```python
from build123d import *

# Parameters (mm, degrees)
CROQUIS1_W                 = 7.5
CROQUIS1_H                 = 6.1
SALIENTE_EXTRUIR2_DEPTH    = 5
CROQUIS2_R                 = 1.6
CORTAR_EXTRUIR1_DEPTH      = 18
REDONDEO1_R                = 1
CORTAR_EXTRUIR2_DEPTH      = 38.482562804
CORTAR_EXTRUIR2_DEPTH_BACK = 38.482562804
CROQUIS3_R                 = 2.1
REDONDEO2_R                = 2


with BuildPart() as part:
    # Croquis1 → Saliente-Extruir2 (new, symmetric)
    # profile 1 of 8: a face of its own
    with BuildSketch(Plane.XY):
        with BuildLine():
            ThreePointArc((12.649110641, 13.5), (6.800735254, 17.204650534), (-1e-09, 18.5))
            ThreePointArc((-1e-09, 18.5), (-6.800735255, 17.204650534), (-12.649110641, 13.5))
            ThreePointArc((-12.649110641, 13.5), (-7.356679045, -16.974371076), (18.5, 0))
            ThreePointArc((18.5, 0), (16.974371076, 7.356679045), (12.649110641, 13.5))
        make_face()
        with BuildLine():
            ThreePointArc((11.05, 0), (-7.813529932, -7.813529932), (0, 11.05))
            ThreePointArc((0, 11.05), (7.813529932, 7.813529932), (11.05, 0))
        make_face(mode=Mode.SUBTRACT)
    # profile 2 of 8: a face of its own
    with BuildSketch(Plane.XY):
        with BuildLine():
            ThreePointArc((12.649110641, 13.5), (6.800735254, 17.204650534), (-1e-09, 18.5))
            ThreePointArc((-1e-09, 18.5), (-6.800735255, 17.204650534), (-12.649110641, 13.5))
            ThreePointArc((-12.649110641, 13.5), (-7.356679045, -16.974371076), (18.5, 0))
            ThreePointArc((18.5, 0), (16.974371076, 7.356679045), (12.649110641, 13.5))
        make_face()
        with BuildLine():
            ThreePointArc((11.05, 0), (-7.813529932, -7.813529932), (0, 11.05))
            ThreePointArc((0, 11.05), (7.813529932, 7.813529932), (11.05, 0))
        make_face(mode=Mode.SUBTRACT)
    # profile 3 of 8: a face of its own
    with BuildSketch(Plane.XY):
        with BuildLine():
            Line((7.5, 18.5), (-1e-09, 18.5))
            ThreePointArc((-1e-09, 18.5), (6.800735254, 17.204650534), (12.649110641, 13.5))
            Line((12.649110641, 13.5), (22.5, 13.5))
            Line((22.5, 13.5), (22.5, 18.5))
            Line((22.5, 18.5), (7.5, 18.5))
        make_face()
    # profile 4 of 8: a face of its own
    with BuildSketch(Plane.XY):
        with BuildLine():
            Line((-7.5, 18.5), (-22.5, 18.5))
            Line((-22.5, 18.5), (-22.5, 13.5))
            Line((-22.5, 13.5), (-12.649110641, 13.5))
            ThreePointArc((-12.649110641, 13.5), (-6.800735255, 17.204650534), (-1e-09, 18.5))
            Line((-1e-09, 18.5), (-7.5, 18.5))
        make_face()
    # profile 5 of 8: a face of its own
    with BuildSketch(Plane.XY):
        Polygon((-22.5, 21.5), (-7.5, 21.5), (-7.5, 24.6), (0, 24.6), (0, 29.558290112), (-22.5, 29.558290112), (-22.5, 24.558290112), align=None)
    # profile 6 of 8: a face of its own
    with BuildSketch(Plane.XY):
        with Locations((3.75, 21.55)):
            Rectangle(CROQUIS1_W, CROQUIS1_H)
    # profile 7 of 8: a face of its own
    with BuildSketch(Plane.XY):
        Polygon((-7.5, 21.5), (-7.5, 18.5), (-1e-09, 18.5), (0, 24.6), (-7.5, 24.6), align=None)
    # profile 8 of 8: a face of its own
    with BuildSketch(Plane.XY):
        Polygon((0, 29.558290112), (0, 24.6), (7.5, 24.6), (22.5, 24.6), (22.5, 29.558290112), align=None)
    extrude(amount=SALIENTE_EXTRUIR2_DEPTH, both=True)

    # Croquis2 → Cortar-Extruir1 (cut)
    with BuildSketch(Plane(origin=(0, 29.558290112, 0), x_dir=(1, 0, 0), z_dir=(0, 1, 0))):
        with Locations(Location((-17.5, 0, 0), (0, 0, 270))):
            Circle(CROQUIS2_R)
        with Locations(Location((17.5, 0, 0), (0, 0, 270))):
            Circle(CROQUIS2_R)
    extrude(amount=-CORTAR_EXTRUIR1_DEPTH, mode=Mode.SUBTRACT)

    # Redondeo1
    redondeo1_edges = [part.edges().sort_by_distance(p)[0] for p in [
        (7.813529932, 7.813529932, 5),
    ]]
    fillet(redondeo1_edges, radius=REDONDEO1_R)

    # Croquis3 → Cortar-Extruir2 (cut, two sides: drawn at the far end of the back side and taken through both)
    with BuildSketch(Plane(origin=(0, 0, 0), x_dir=(0, 0, -1), z_dir=(1, 0, 0)).offset(-CORTAR_EXTRUIR2_DEPTH_BACK)):
        Circle(CROQUIS3_R)
    extrude(amount=CORTAR_EXTRUIR2_DEPTH + CORTAR_EXTRUIR2_DEPTH_BACK, mode=Mode.SUBTRACT)

    # Redondeo2
    redondeo2_edges = [part.edges().sort_by_distance(p)[0] for p in [
        (22.5, 16, -5),
        (-22.5, 16, -5),
        (-22.5, 25.529145056, -5),
        (22.5, 27.079145056, 5),
        (22.5, 27.079145056, -5),
        (-22.5, 25.529145056, 5),
        (-22.5, 16, 5),
        (22.5, 16, 5),
    ]]
    fillet(redondeo2_edges, radius=REDONDEO2_R)


solid = part.part
```
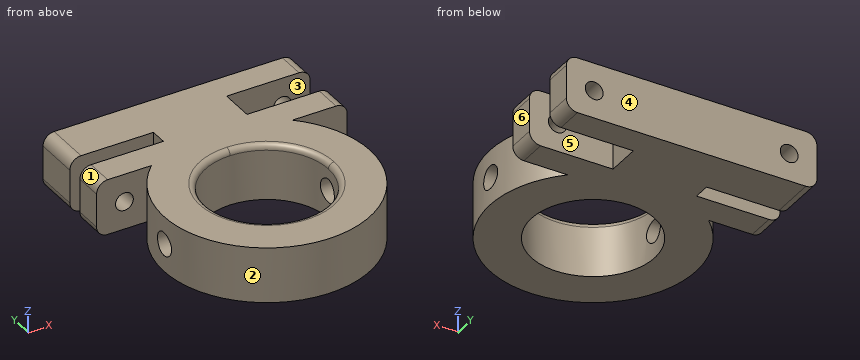
CAD build for the part. Positions are in the model's coordinates, mm. Face numbers are marked on the shaded views. A direction names the side the tool comes from. Give positions to 0.01 mm unless a question says otherwise; leave off trailing zeros. Loops run counter-clockwise (first coordinate to the right, second up) from the corner with the lowest first, then second, coordinate; pieces in that order, holes last. Notation, with made-up numbers: (13, 14) -> (41, 14) arc R18 ccw to (41, 32) -> close; hole circle Ø2 at (81, 67.25). An arc over 180 degrees is marked (long way). Use a Markdown table: item, result.
1. Flat gauge pins, fed straight in: pin 1 (3 mm diameter, centred on y = 22, z = -0.5, fed in from +X); pin 2 (1.5 mm diameter, centred on y = 19.5, z = -2, fed in from -X); pin 3 (5.5 mm diameter, centred on y = 0, z = 0, fed in from +X). Where does each tip first touch, or does it go through?
Check result:
| item | result |
|---|---|
| pin 1 | stops at x = 7.5 |
| pin 2 | stops at x = -7.5 |
| pin 3 | stops at x = 18.5 |
2. Slice it at D-D (z = -1). Give the number of separate pieces and of enclosed holes in the cut face, plus the area to 3 significant figures.
Check result:
| item | result |
|---|---|
| separate pieces | 6 |
| enclosed holes | 0 |
| area | 1,080 mm^2 |
3. Wall check: L1, parallel to Y at x = -13.5, z = 0; L2, parallel to X at y = 16, z = 1; L3, parallel to Y at x = 16, z = 1.5. Give the ranges that are in metal, low to high. Write a range as [from, to].
Check result:
| item | result |
|---|---|
| L1 | y = [-12.65, -2.1], [2.1, 12.65], [13.5, 18.5], [21.5, 29.56] |
| L2 | x = [-22.5, -18.75], [-16.25, 16.25], [18.75, 22.5] |
| L3 | y = [-9.29, -1.47], [1.47, 9.29], [13.5, 18.5], [24.6, 29.56] |
4. Mould opens along Y. For the marked faces 1, 2, 3 and 4 say: pulls with the +Y half, pulls with the -Y half, needs draft (parallel to the pull), parting line crosses it, or undercut.
Check result:
| item | result |
|---|---|
| face 1 | needs draft |
| face 2 | undercut |
| face 3 | undercut |
| face 4 | pulls with the +Y half |
5. Slice it at B-B (x = 17.5). List the corners of the cut face in (y, z).
Check result:
| item | result |
|---|---|
| outline | (-6, -5) -> (6, -5) -> (6, 5) -> (-6, 5) -> close; (13.5, -5) -> (18.5, -5) -> (18.5, -1.6) -> (13.5, -1.6) -> close; (13.5, 1.6) -> (18.5, 1.6) -> (18.5, 5) -> (13.5, 5) -> close; (24.6, -5) -> (29.56, -5) -> (29.56, -1.6) -> (24.6, -1.6) -> close; (24.6, 1.6) -> (29.56, 1.6) -> (29.56, 5) -> (24.6, 5) -> close; hole circle Ø4.2 at (0, 0) |
6. Slice it at C-C (y = 20). List the corners of the cut face in (x, z).
Check result:
| item | result |
|---|---|
| outline | (-7.5, -5) -> (7.5, -5) -> (7.5, 5) -> (-7.5, 5) -> close |
7. Which spindle directions (+Z, -Z, +X, -X, +Y, -Y) get a long thin tool onto all of the face, cutting with end or side? Do the marked faces 5 and 6. Say none if no direction does.
Check result:
| item | result |
|---|---|
| face 5 | +Z, -Z, +X |
| face 6 | +Z, -Z, +X, +Y, -Y |
8. Slice it at A-A (x = -13.5). List the corners of the cut face in (y, z).
Check result:
| item | result |
|---|---|
| outline | (-12.65, -5) -> (12.65, -5) -> (12.65, 5) -> (-12.65, 5) -> close; (13.5, -5) -> (18.5, -5) -> (18.5, 5) -> (13.5, 5) -> close; (21.5, -5) -> (29.56, -5) -> (29.56, 5) -> (21.5, 5) -> close; hole circle Ø4.2 at (0, 0) |
